Geometry check sheet. Reference: drawing and pictorial views, mm from the part's lowest x, y, z. Round coordinates to 2 decimals unless told otherwise and drop trailing zeros. Order: outer loops, then holes, each group sorted by start corner. A loop starts at its lowest first (then second) coordinate and runs counter-clockwise, first axis right, second up.
(1) Sectioned sample at B-B (z = 45). Record the boundary of the cut face in (x, y).
(2) Sectioned sample at A-A (x = 225). Record the boundary of the cut face in (y, z), plus the area to 3 significant figures.
(3) Go/stop test with flat-tipped pins: pin 1 (4 mm diameter, centred on x = 135.59, z = 30.91, fed in from -Y); pin 2 (4.5 mm diameter, centred on x = 148, z = 10, fed in from +Y); pin 3 (1.5 mm diameter, centred on x = 148.5, y = 4, fed in from -Z). Record where each tip stops, or that it passes through.
(4) Material ranges on line 1 along Z through (x, y) = (225, 3.3); line 2 along X through (y, z) = (1.8, 58); line 3 along X through (y, z) = (3.9, 10), recorded low to high.
(5) Sectioned sample at D-D (z = 4.5). Record the boundary of the cut face in (x, y).
(6) Sectioned sample at C-C (y = 2.8). Give the number of separate pieces and of enclosed holes in the cut face, plus the area to 3 significant figures.
(7) Release check for a two-part mould opening along X. For the marked faces 1 and 2 record: +X half, -X half, draft (parallel to the pull), parting line (faces both ways), or undercut.
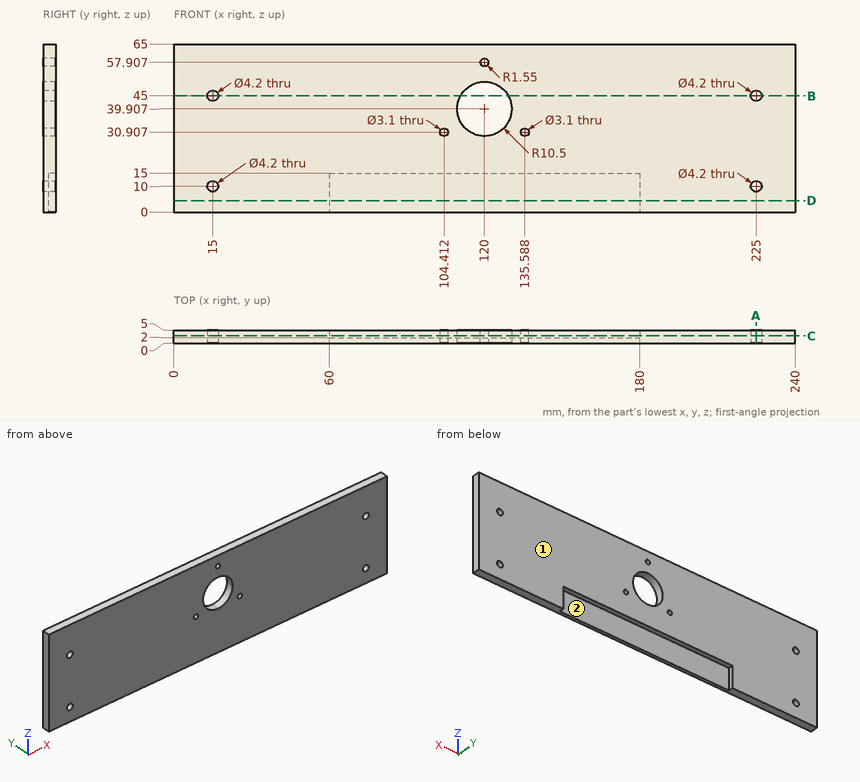
Answer below:
1. outline: (0, 0) - (12.9, 0) - (12.9, 5) - (0, 5) - close; (17.1, 0) - (110.82, 0) - (110.82, 5) - (17.1, 5) - close; (129.18, 0) - (222.9, 0) - (222.9, 5) - (129.18, 5) - close; (227.1, 0) - (240, 0) - (240, 5) - (227.1, 5) - close
2. outline: (0, 0) - (5, 0) - (5, 7.9) - (0, 7.9) - close; (0, 12.1) - (5, 12.1) - (5, 42.9) - (0, 42.9) - close; (0, 47.1) - (5, 47.1) - (5, 65) - (0, 65) - close
2. area: 283 mm2
3. pin 1: stops at y = 0
3. pin 2: stops at y = 2
3. pin 3: stops at z = 15
4. line 1: z = 0 to 7.9, 12.1 to 42.9, 47.1 to 65
4. line 2: x = 0 to 118.45, 121.55 to 240
4. line 3: x = 0 to 12.9, 17.1 to 60, 180 to 222.9, 227.1 to 240
5. outline: (0, 0) - (240, 0) - (240, 5) - (180, 5) - (180, 2) - (60, 2) - (60, 5) - (0, 5) - close
6. separate pieces: 1
6. enclosed holes: 8
6. area: 13,400 mm2
7. face 1: draft
7. face 2: undercut
